The figure shows three views and two pictorial views of one solid part (mm, origin at its lowest corner). Answer the questions. Coordinates: 2 decimals unless noted, no trailing zeros. Order: outer loops, then holes, each group sorted by start corner. A loop starts at its lowest first (then second) coordinate and runs counter-clockwise, first axis right, second up. Notation, with made-up numbers: M 28,72 L 60,72 A22 ccw 60,84 Z; hole C 1.5,78.25 d6. An arc over 180 degrees is marked long. Answer in a Markdown table with one row per item. Add a question column.
Item 1: The part is cut by section B-B (y = 3.9). Write down the section's boundary in (x, z).
Item 2: The mould has two halves that part along X. Classify the marked faces 1, 2 and 3: released by +X, released by -X, zero draft, split by the parting line, or undercut.
Item 3: The part is cut by section C-C (x = 7). Write down the section's boundary in (y, z), then the cut area to 3 significant figures.
Item 4: The part is cut by section D-D (x = 9). Write down the section's boundary in (y, z).
Item 5: The part is cut by section A-A (x = 5). Write down the section's boundary in (y, z), then the cut area to 3 significant figures.
Item 6: Consider line 1 (Z direction, x = 5, y = 2.7); line 2 (Z direction, x = 3.5, y = 3.05); line 3 (Z direction, x = 8, y = 3.1). Determine where each line is inside the solid, lowest interval first. Write a range as from..to.
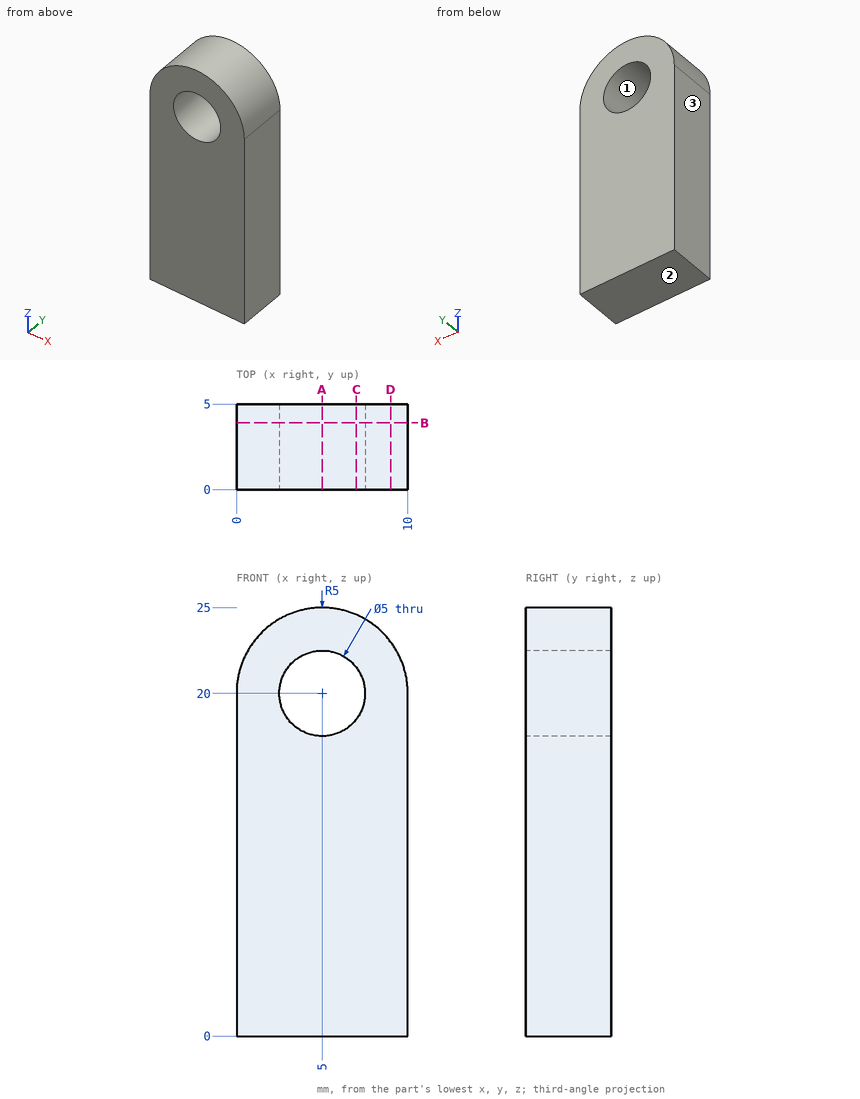
Reply:
| question | item | result |
|---|---|---|
| 1 | outline | M 0,0 L 10,0 L 10,20 A5 ccw 0,20 Z; hole C 5,20 d5 |
| 2 | face 1 | undercut |
| 2 | face 2 | zero draft |
| 2 | face 3 | released by -X |
| 3 | outline | M 0,0 L 5,0 L 5,18.5 L 0,18.5 Z; M 0,21.5 L 5,21.5 L 5,24.58 L 0,24.58 Z |
| 3 | area | 108 mm2 |
| 4 | outline | M 0,0 L 5,0 L 5,23 L 0,23 Z |
| 5 | outline | M 0,0 L 5,0 L 5,17.5 L 0,17.5 Z; M 0,22.5 L 5,22.5 L 5,25 L 0,25 Z |
| 5 | area | 100 mm2 |
| 6 | line 1 | z = 0..17.5, 22.5..25 |
| 6 | line 2 | z = 0..18, 22..24.77 |
| 6 | line 3 | z = 0..24 |
